Part print with two shaded views. Sizes in mm from the minimum x, y, z corner. A direction names the side the tool comes from. Round coordinates to 2 decimals unless told otherwise and drop trailing zeros. Write each loop counter-clockwise with the first axis right and the second up, starting at its lowest first coordinate (ties: lowest second). Pieces come first, ordered by that corner, then holes. Notation, with made-up numbers: (-14.75, 45) -> (2.25, 45) arc R22 ccw to (2.25, 83) -> close; hole circle Ø9 at (61, -11). An arc over 180 degrees is marked (long way). Return JSON: item names as keys, results as strings.
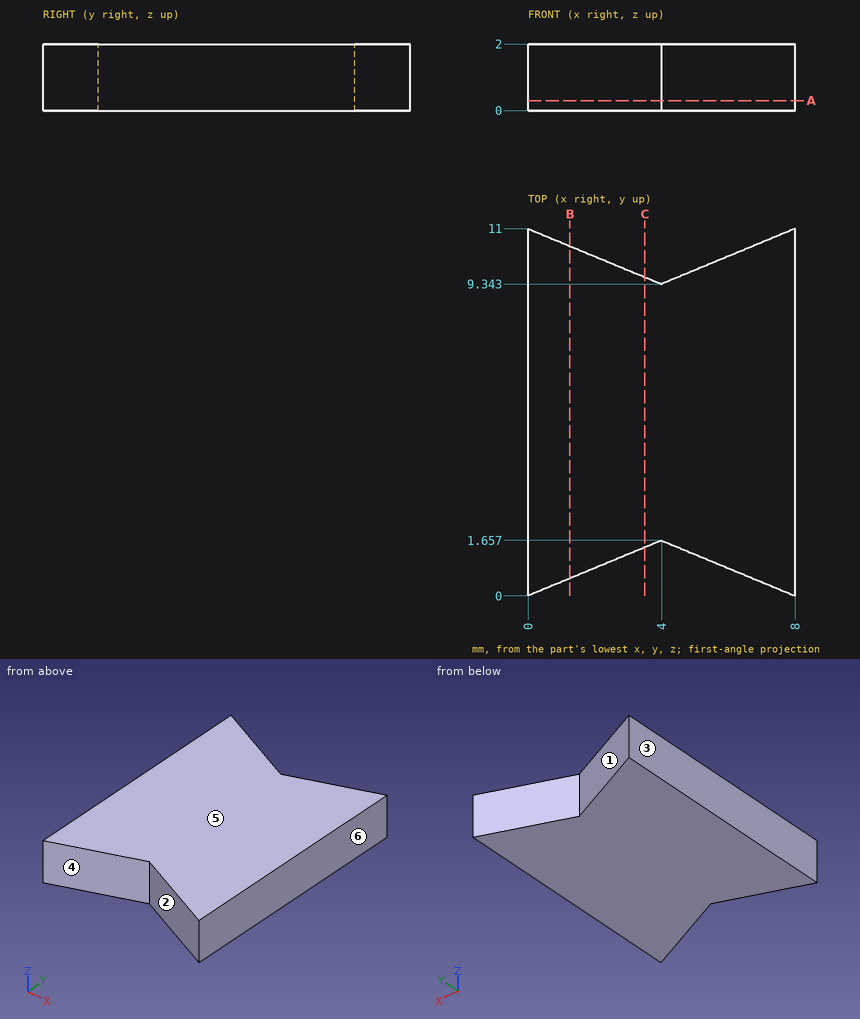
Q1. 3-axis set-ups, long thin cutter, end or side, ignore diameter. For the marked faces 1, 2 and 3: which of +Z, -Z, +X, -X, +Y, -Y reach the whole face in a straight line?
Verdict:
{"face 1": "+Z, -Z, +Y", "face 2": "+Z, -Z, -Y", "face 3": "+Z, -Z, -X, +Y, -Y"}
Q2. Two-plate mould, pull along X, no slides. Class the marked faces 4, 5 and 6: +X half, -X half, draft (parallel to the pull), parting line (faces both ways), or undercut.
Verdict:
{"face 4": "undercut", "face 5": "draft", "face 6": "+X half"}
Q3. Saw through at A-A on z = 0.3. List the corners of the cut face in (x, y).
Verdict:
{"outline": "(0, 0) -> (4, 1.66) -> (8, 0) -> (8, 11) -> (4, 9.34) -> (0, 11) -> close"}
Q4. Wall check: L1, parallel to X at y = 1, z = 0.25 (1 decimal); L2, parallel to X at y = 10.25, z = 1.3; L3, parallel to Y at x = 2.75, z = 0.3. Give the ranges that are in metal, low to high.
Verdict:
{"L1": "x = 0 to 2.4, 5.6 to 8", "L2": "x = 0 to 1.81, 6.19 to 8", "L3": "y = 1.14 to 9.86"}
Q5. Saw through at B-B on x = 1.25. List the corners of the cut face in (y, z), then the cut area to 3 significant figures.
Verdict:
{"outline": "(0.52, 0) -> (10.48, 0) -> (10.48, 2) -> (0.52, 2) -> close", "area": "19.9 mm²"}
Q6. Saw through at C-C on x = 3.5. List the corners of the cut face in (y, z), then the cut area to 3 significant figures.
Verdict:
{"outline": "(1.45, 0) -> (9.55, 0) -> (9.55, 2) -> (1.45, 2) -> close", "area": "16.2 mm²"}
